Design review of the part built by this model. Coordinates are the model's own, in mm. A direction names the side the tool comes from. Coordinates: 2 decimals unless noted, no trailing zeros. Write each loop counter-clockwise with the first axis right and the second up, starting at its lowest first coordinate (ties: lowest second). Pieces come first, ordered by that corner, then holes. Notation, with made-up numbers: (-15, 7.5) -> (22, 7.5) arc R35 ccw to (22, 44.5) -> close; hole circle Ø7 at (28.5, 44). An arc over 180 degrees is marked (long way). Answer in a Markdown table with one row per item. Add a question column.
Item 1: To check wall thickness, follow line 1 (X direction, y = 88, z = -139.5); line 2 (X direction, y = 17.5, z = -123); line 3 (X direction, y = 55, z = -44). State the ranges of each line that lie inside material, in increasing order.
Item 2: Take a section at B-B, the plane z = -16.5. Write out the cut boundary in (x, y).
Item 3: Take a section at A-A, the plane y = 72.5. Write out the cut boundary in (x, z), and give its area (3 significant figures).
Item 4: Take a section at C-C, the plane x = 224.5. Write out the cut boundary in (y, z).
Item 5: For faces 3 (the face through (25, 54, -50)), 4 (the face through (325, 100, -125)), 5 (the face through (100, 30, -25)), list the 3-axis set-ups (+Z, -Z, +X, -X, +Y, -Y) from which the entire face can be reached by the end or side of a thin tool; tool diameter is ignored.
Item 6: Draft analysis for pull direction X (two halves, no side actions). For faces 1 (the face through (325, 30, -50)), 2 (the face through (400, 30, -125)), state which applies: released by +X, released by -X, zero draft, split by the parting line, or undercut.
Item 7: Clearance check with flat-ended pins moving along their axes: P1, Ø1.5, axis at x = 389.5, z = -127, coming from the +Y side; P2, Ø15, axis at x = 220.5, y = 77.5, coming from the +Z side; P3, Ø15, axis at y = 76.5, z = -115.5, coming from the +X side. State where each tip first meets the part, or that it passes through.
Item 8: Take a section at D-D, the plane y = 44.5. Give the number of separate pieces and of enclosed holes in the cut face, and give its area (3 significant figures).
from build123d import *

# Parameters (mm, degrees)
BOSS_EXTRUDE3_DEPTH = 10
SKETCH2_5_W         = 50
SKETCH2_5_H         = 50
BOSS_EXTRUDE4_DEPTH = 100
SKETCH2_6_W         = 50
SKETCH2_6_H         = 50
BOSS_EXTRUDE5_DEPTH = 50


with BuildPart() as part:
    # Sketch2 → Boss-Extrude3 (new body)
    with BuildSketch(Plane(origin=(0, 0, 0), x_dir=(1, 0, 0), z_dir=(0, 1, 0))):
        Polygon((450, 75), (0, 75), (0, 50), (50, 50), (50, 0), (100, 0), (100, 50), (150, 50), (150, 0), (200, 0), (200, 50), (250, 50), (250, 0), (300, 0), (300, 50), (350, 50), (350, 0), (400, 0), (400, 50), (450, 50), align=None)
        Polygon((100, 100), (100, 150), (50, 150), (50, 100), (0, 100), (0, 75), (450, 75), (450, 100), (400, 100), (400, 150), (350, 150), (350, 100), (300, 100), (300, 150), (250, 150), (250, 100), (200, 100), (200, 150), (150, 150), (150, 100), align=None)
    extrude(amount=BOSS_EXTRUDE3_DEPTH)

    # Sketch2_5 → Boss-Extrude4 (add)
    with BuildSketch(Plane(origin=(0, 0, 0), x_dir=(1, 0, 0), z_dir=(0, 1, 0))):
        with Locations((25, 25)):
            Rectangle(SKETCH2_5_W, SKETCH2_5_H)
        with Locations((125, 125)):
            Rectangle(SKETCH2_5_W, SKETCH2_5_H)
        with Locations((225, 125)):
            Rectangle(SKETCH2_5_W, SKETCH2_5_H)
        with Locations((325, 125)):
            Rectangle(SKETCH2_5_W, SKETCH2_5_H)
        with Locations((425, 25)):
            Rectangle(SKETCH2_5_W, SKETCH2_5_H)
    extrude(amount=BOSS_EXTRUDE4_DEPTH)

    # Sketch2_6 → Boss-Extrude5 (add)
    with BuildSketch(Plane(origin=(0, 0, 0), x_dir=(1, 0, 0), z_dir=(0, 1, 0))):
        with Locations((25, 125)):
            Rectangle(SKETCH2_6_W, SKETCH2_6_H)
        with Locations((125, 25)):
            Rectangle(SKETCH2_6_W, SKETCH2_6_H)
        with Locations((425, 125)):
            Rectangle(SKETCH2_6_W, SKETCH2_6_H)
        with Locations((225, 25)):
            Rectangle(SKETCH2_6_W, SKETCH2_6_H)
        with Locations((325, 25)):
            Rectangle(SKETCH2_6_W, SKETCH2_6_H)
    extrude(amount=BOSS_EXTRUDE5_DEPTH)


solid = part.part
Answers:
| question | item | result |
|---|---|---|
| 1 | line 1 | x = 100 to 150, 200 to 250, 300 to 350 |
| 1 | line 2 | x = 0 to 50, 100 to 150, 200 to 250, 300 to 350, 400 to 450 |
| 1 | line 3 | x = 0 to 50, 400 to 450 |
| 2 | outline | (0, 0) -> (450, 0) -> (450, 100) -> (400, 100) -> (400, 10) -> (350, 10) -> (350, 50) -> (300, 50) -> (300, 10) -> (250, 10) -> (250, 50) -> (200, 50) -> (200, 10) -> (150, 10) -> (150, 50) -> (100, 50) -> (100, 10) -> (50, 10) -> (50, 100) -> (0, 100) -> close |
| 3 | outline | (0, -50) -> (50, -50) -> (50, 0) -> (0, 0) -> close; (100, -150) -> (150, -150) -> (150, -100) -> (100, -100) -> close; (200, -150) -> (250, -150) -> (250, -100) -> (200, -100) -> close; (300, -150) -> (350, -150) -> (350, -100) -> (300, -100) -> close; (400, -50) -> (450, -50) -> (450, 0) -> (400, 0) -> close |
| 3 | area | 12,500 mm^2 |
| 4 | outline | (0, -150) -> (100, -150) -> (100, -100) -> (10, -100) -> (10, -50) -> (50, -50) -> (50, 0) -> (0, 0) -> close |
| 5 | face 3 | +X, -X, +Y |
| 5 | face 4 | +Z, -Z, +X, -X, +Y |
| 5 | face 5 | +Z, -Z, +Y |
| 6 | face 1 | zero draft |
| 6 | face 2 | undercut |
| 7 | P1 | stops at y = 10 |
| 7 | P2 | stops at z = -100 |
| 7 | P3 | stops at x = 350 |
| 8 | separate pieces | 10 |
| 8 | enclosed holes | 0 |
| 8 | area | 25,000 mm^2 |
